Input: part model. Units: mm. Frame: model coordinates. A direction names the side the tool comes from. Round coordinates to 2 decimals unless told otherwise and drop trailing zeros. Loops run counter-clockwise (first coordinate to the right, second up) from the corner with the lowest first, then second, coordinate; pieces in that order, holes last. Notation, with made-up numbers: M 53.5,39.25 L 86.5,39.25 A14 ccw 86.5,55.25 Z; hole C 50.5,88 d8. An arc over 180 degrees is marked long. Use one line per item in the form item = value. Start each with the question number.
Q1. First-contact query: P1, Ø10, axis at y = 12, z = -372.5, coming from the -X side; P2, Ø1, axis at y = 23.5, z = -90.5, coming from the -X side; P3, Ø4, axis at x = -301.5, y = -46.5, coming from the +Z side. Flat tips, straight axial feed; report the tip coordinate or a pass-through.
Q2. Access query for faces 1 (the cylindrical face through (148.148, 2.1, 144.523)), 2 (the flat face through (55.102, -2.1, -295.396)). Directions: +Z, -Z, +X, -X, +Y, -Y. A direction counts if a zero-diameter tool reaches every point of the face in a straight line with its end or side. Return the directions, or none.
Q3. Section query C-C, the plane x = 32.5. Output: boundary loops of the cut face in (y, z), and give its area (3 significant figures).
Q4. Mould query, pull axis Z, two halves, no side actions, for faces 3 (the flat face through (54, 150, -56)), 4 (the flat face through (-54.222, 2.1, -296.204)), 5 (the flat face through (272, 2, 28)). Classes: pulls with the +Z half, pulls with the -Z half, needs draft (parallel to the pull), parting line crosses it, or undercut.
Q5. Section query D-D, the plane z = 14.5. Output: boundary loops of the cut face in (x, y), and give its area (3 significant figures).
Q6. Section query B-B, the plane x = -275. Output: boundary loops of the cut face in (y, z).
Q7. Section query A-A, the plane z = -128.5. Output: boundary loops of the cut face in (x, y), and give its area (3 significant figures).
Q8. Ray query, line 1 along X through (y, z) = (47.5, -232.5); line 2 along X through (y, z) = (122.5, -18.5); line 3 along Z through (x, y) = (-82, 33). Return the intervals inside material, ascending.
```python
from build123d import *

# Parameters (mm, degrees)
F0_R     = 50
F1_DEPTH = 150


# Not quite as in the source:
# - a feature names something its author has since deleted; it is built from what else it names


with BuildPart() as f1:
    # F0 (on Front) → F1 (new body, symmetric)
    with BuildSketch(Plane.XZ):
        with BuildLine():
            Line((-170.5025253169, 129.4974746831), (-300, 0))
            Line((-300, 0), (-292.9289321881, -7.0710678119))
            Line((-292.9289321881, -7.0710678119), (-285.8578643763, 0))
            Line((-285.8578643763, 0), (-166.3603896932, 119.4974746831))
            ThreePointArc((-166.3603896932, 119.4974746831), (-143.6507552757, 134.6715672758), (-116.8629150102, 140))
            Line((-116.8629150102, 140), (116.8629150102, 140))
            ThreePointArc((116.8629150102, 140), (143.6507552757, 134.6715672758), (166.3603896932, 119.4974746831))
            Line((166.3603896932, 119.4974746831), (285.8578643763, 0))
            Line((285.8578643763, 0), (292.9289321881, -7.0710678119))
            Line((292.9289321881, -7.0710678119), (150, -150))
            Line((150, -150), (59.5836943966, -240.4163056034))
            Line((59.5836943966, -240.4163056034), (86.0845268471, -266.917138054))
            Line((86.0845268471, -266.917138054), (121.4712095943, -302.3038208012))
            Line((121.4712095943, -302.3038208012), (130.2943725152, -311.1269837221))
            ThreePointArc((130.2943725152, -311.1269837221), (147.9720420449, -318.4493141924), (165.6497115746, -311.1269837221))
            Line((165.6497115746, -311.1269837221), (370.7106781187, -106.066017178))
            ThreePointArc((370.7106781187, -106.066017178), (378.033008589, -88.3883476483), (370.7106781187, -70.7106781187))
            Line((370.7106781187, -70.7106781187), (300, 0))
            Line((300, 0), (170.5025253169, 129.4974746831))
            ThreePointArc((170.5025253169, 129.4974746831), (147.7928908994, 144.6715672758), (121.0050506339, 150))
            Line((121.0050506339, 150), (-121.0050506339, 150))
            ThreePointArc((-121.0050506339, 150), (-147.7928908994, 144.6715672758), (-170.5025253169, 129.4974746831))
        make_face()
        with BuildLine():
            Line((73.7258300203, -240.4163056034), (300, -14.1421356237))
            Line((300, -14.1421356237), (356.5685424949, -70.7106781187))
            ThreePointArc((356.5685424949, -70.7106781187), (363.8908729653, -88.3883476483), (356.5685424949, -106.066017178))
            Line((356.5685424949, -106.066017178), (165.6497115746, -296.9848480984))
            ThreePointArc((165.6497115746, -296.9848480984), (147.9720420449, -304.3071785687), (130.2943725152, -296.9848480984))
            Line((130.2943725152, -296.9848480984), (73.7258300203, -240.4163056034))
        make_face(mode=Mode.SUBTRACT)
        with BuildLine():
            Line((-17.6776695297, -17.6776695297), (-150, -150))
            Line((-150, -150), (-59.5836943966, -240.4163056034))
            Line((-59.5836943966, -240.4163056034), (-17.6776695297, -282.3223304703))
            ThreePointArc((-17.6776695297, -282.3223304703), (0, -289.6446609407), (17.6776695297, -282.3223304703))
            Line((17.6776695297, -282.3223304703), (59.5836943966, -240.4163056034))
            Line((59.5836943966, -240.4163056034), (150, -150))
            Line((150, -150), (17.6776695297, -17.6776695297))
            ThreePointArc((17.6776695297, -17.6776695297), (0, -10.3553390593), (-17.6776695297, -17.6776695297))
        make_face()
        with BuildLine():
            ThreePointArc((17.6776695297, -268.1801948466), (0, -275.5025253169), (-17.6776695297, -268.1801948466))
            Line((-17.6776695297, -268.1801948466), (-125.8578643763, -160))
            Line((-125.8578643763, -160), (-135.8578643763, -150))
            Line((-135.8578643763, -150), (-67.9289321881, -82.0710678119))
            Line((-67.9289321881, -82.0710678119), (-17.6776695297, -31.8198051534))
            ThreePointArc((-17.6776695297, -31.8198051534), (0, -24.4974746831), (17.6776695297, -31.8198051534))
            Line((17.6776695297, -31.8198051534), (67.9289321881, -82.0710678119))
            Line((67.9289321881, -82.0710678119), (135.8578643763, -150))
            Line((135.8578643763, -150), (125.8578643763, -160))
            Line((125.8578643763, -160), (17.6776695297, -268.1801948466))
        make_face(mode=Mode.SUBTRACT)
        with BuildLine():
            Line((-292.9289321881, -7.0710678119), (-300, 0))
            Line((-300, 0), (-370.7106781187, -70.7106781187))
            ThreePointArc((-370.7106781187, -70.7106781187), (-378.033008589, -88.3883476483), (-370.7106781187, -106.066017178))
            Line((-370.7106781187, -106.066017178), (-165.6497115746, -311.1269837221))
            ThreePointArc((-165.6497115746, -311.1269837221), (-147.9720420449, -318.4493141924), (-130.2943725152, -311.1269837221))
            Line((-130.2943725152, -311.1269837221), (-121.4712095523, -302.3038207591))
            Line((-121.4712095523, -302.3038207591), (-86.0845268892, -266.917138096))
            Line((-86.0845268892, -266.917138096), (-59.5836943966, -240.4163056034))
            Line((-59.5836943966, -240.4163056034), (-150, -150))
            Line((-150, -150), (-292.9289321881, -7.0710678119))
        make_face()
        with BuildLine():
            Line((-356.5685424949, -70.7106781187), (-300, -14.1421356237))
            Line((-300, -14.1421356237), (-73.7258300203, -240.4163056034))
            Line((-73.7258300203, -240.4163056034), (-130.2943725152, -296.9848480984))
            ThreePointArc((-130.2943725152, -296.9848480984), (-147.9720420449, -304.3071785687), (-165.6497115746, -296.9848480984))
            Line((-165.6497115746, -296.9848480984), (-356.5685424949, -106.066017178))
            ThreePointArc((-356.5685424949, -106.066017178), (-363.8908729653, -88.3883476483), (-356.5685424949, -70.7106781187))
        make_face(mode=Mode.SUBTRACT)
        with BuildLine():
            ThreePointArc((23.2387555319, -324.683089695), (-4.1825e-06, -319.9999946001), (-23.238764161, -324.6830883841))
            ThreePointArc((-23.238764161, -324.6830883841), (-44.1741271353, -339.3964601375), (-57.0750428799, -361.4948561013))
            ThreePointArc((-57.0750428799, -361.4948561013), (-9.3674436165, -439.2642427617), (59.9999941253, -379.9999946001))
            ThreePointArc((59.9999941253, -379.9999946001), (59.264242551, -370.6325585299), (57.0750321743, -361.4948593208))
            ThreePointArc((57.0750321743, -361.4948593208), (44.1741176762, -339.3964626293), (23.2387555319, -324.683089695))
        make_face()
        with Locations((-5.8747e-06, -379.9999946001)):
            Circle(F0_R, mode=Mode.SUBTRACT)
        with BuildLine():
            Line((86.0845268471, -266.917138054), (23.2387555319, -324.683089695))
            ThreePointArc((23.2387555319, -324.683089695), (44.1741176762, -339.3964626293), (57.0750321743, -361.4948593208))
            Line((57.0750321743, -361.4948593208), (121.4712095943, -302.3038208012))
            Line((121.4712095943, -302.3038208012), (86.0845268471, -266.917138054))
        make_face()
        with BuildLine():
            Line((-23.238764161, -324.6830883841), (-86.0845268892, -266.917138096))
            Line((-86.0845268892, -266.917138096), (-121.4712095523, -302.3038207591))
            Line((-121.4712095523, -302.3038207591), (-57.0750428799, -361.4948561013))
            ThreePointArc((-57.0750428799, -361.4948561013), (-44.1741271353, -339.3964601375), (-23.238764161, -324.6830883841))
        make_face()
        Polygon((-135.8578643763, -150), (-125.8578643763, -160), (125.8578643763, -160), (135.8578643763, -150), align=None)
    extrude(amount=F1_DEPTH, both=True)


solid = f1.part
```
Results found:
q1.P1 = -59.95
q1.P2 = -377.98
q1.P3 = 0.5
q2.face_1 = +Z, +X, +Y, -Y
q2.face_2 = +Y, -Y
q3.outline = M -150,-430.44 L 150,-430.44 L 150,-418 L -150,-418 Z; M -150,-342 L 150,-342 L 150,-316.17 L -150,-316.17 Z; M -150,-267.5 L 150,-267.5 L 150,-253.36 L -150,-253.36 Z; M -150,-160 L 150,-160 L 150,-150 L -150,-150 Z; M -150,-46.64 L 150,-46.64 L 150,-32.5 L -150,-32.5 Z; M -150,140 L 150,140 L 150,150 L -150,150 Z
q3.area = 26,000 mm²
q4.face_3 = needs draft
q4.face_4 = undercut
q4.face_5 = pulls with the +Z half
q5.outline = M -285.5,-150 L -271.36,-150 L -271.36,150 L -285.5,150 Z; M 271.36,-150 L 285.5,-150 L 285.5,150 L 271.36,150 Z
q5.area = 8,490 mm²
q6.outline = M -150,-201.78 L 150,-201.78 L 150,-187.63 L -150,-187.63 Z; M -150,-39.14 L 150,-39.14 L 150,-25 L -150,-25 Z; M -150,10.86 L 150,10.86 L 150,25 L -150,25 Z
q7.outline = M -348.28,-150 L -334.13,-150 L -334.13,150 L -348.28,150 Z; M -185.64,-150 L -171.5,-150 L -171.5,150 L -185.64,150 Z; M -128.5,-150 L -114.36,-150 L -114.36,150 L -128.5,150 Z; M 114.36,-150 L 128.5,-150 L 128.5,150 L 114.36,150 Z; M 171.5,-150 L 185.64,-150 L 185.64,150 L 171.5,150 Z; M 334.13,-150 L 348.28,-150 L 348.28,150 L 334.13,150 Z
q7.area = 25,500 mm²
q8.line_1 = -244.28 to -230.13, -81.64 to -53.36, 53.36 to 81.64, 230.13 to 244.28
q8.line_2 = -318.5 to -304.36, -295.64 to -281.5, -18.5 to 18.5, 281.5 to 295.64, 304.36 to 318.5
q8.line_3 = -338.58 to -270.67, -262.83 to -248.69, -232.14 to -203.86, -160 to -150, -96.14 to -82, 140 to 150
